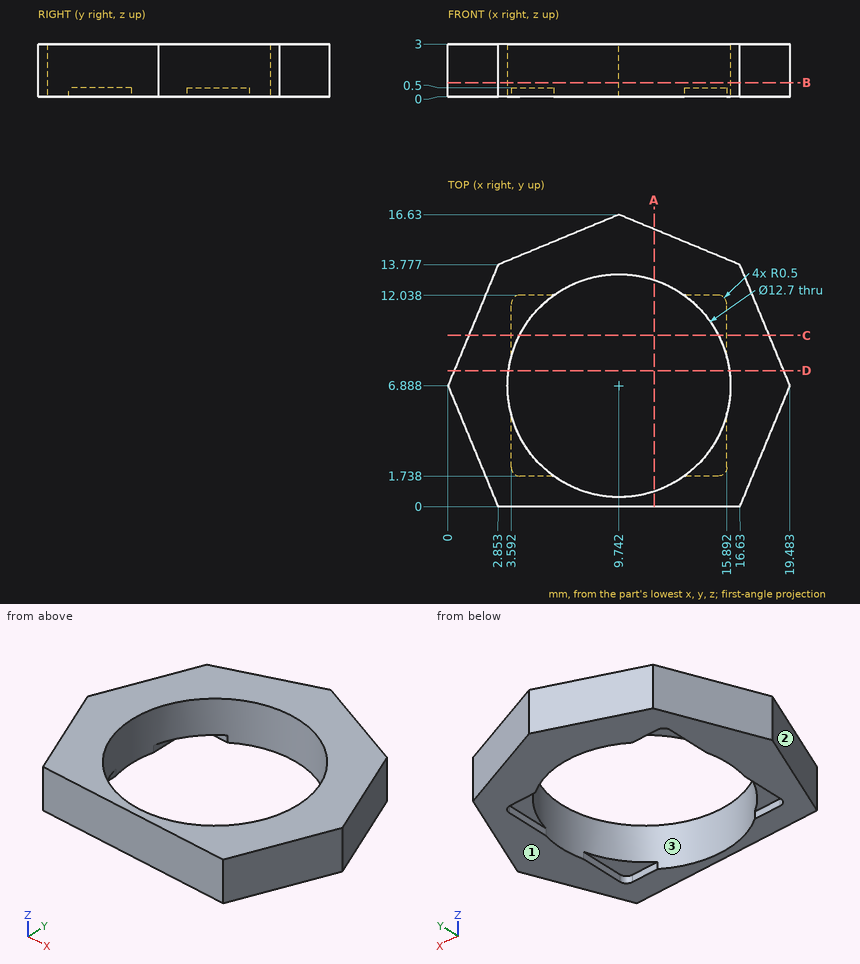
For this review, use the dimensioned drawing (mm, ordinates from the lowest corner) and the shaded views. Give positions to 0.01 mm unless a question says otherwise; leave off trailing zeros. Write each loop counter-clockwise with the first axis right and the second up, starting at its lowest first coordinate (ties: lowest second). Pieces come first, ordered by that corner, then holes. Notation, with made-up numbers: M 46,54.25 L 70,54.25 A8 cw 70,63.25 Z; hole C 45,42.25 d4. An arc over 180 degrees is marked long. Write item = value, one per line. Start each with the question number.
Q1. We need section A-A (x = 11.75). State the section outline as (y, z) points (1 decimal).
Q2. Mouldability with a two-part tool opening along X and no side actions: class the marked faces 1, 2 and 3 as released by +X, released by -X, zero draft, split by the parting line, or undercut.
Q3. For line 1 (X direction, y = 10.5, z = 0.1) (1 decimal); line 2 (X direction, y = 10.25, z = 0.65) (1 decimal); line 3 (Y direction, x = 14.5, z = 1.3) (1 decimal), list the stretches that pass through material, from the lowest coordinate up.
Q4. Clearance check with flat-ended pins moving along their axes: pin 1 (0.7 mm diameter, centred on x = 15, y = 10.5, fed in from -Z); pin 2 (0.6 mm diameter, centred on y = 3.5, z = 0.5, fed in from +X); pin 3 (0.6 mm diameter, centred on x = 5.5, z = 0.5, fed in from +Y). State where each tip first meets the part, or that it passes through.
Q5. We need section D-D (y = 7.75). State the section outline as (x, z) points.
Q6. We need section C-C (y = 9.75). State the section outline as (x, z) points (1 decimal).
Q7. We need section B-B (z = 0.8). State the section outline as (x, y) points, plus the area to 3 significant figures.
Result set:
q1.outline = M 0,0 L 0.9,0 L 0.9,3 L 0,3 Z; M 12.9,0 L 15.8,0 L 15.8,3 L 12.9,3 Z
q2.face_1 = zero draft
q2.face_2 = released by -X
q2.face_3 = undercut
q3.line_1 = 1.5 to 3.6, 15.9 to 18
q3.line_2 = 1.4 to 4.4, 15.1 to 18.1
q3.line_3 = 0 to 2.7, 11.1 to 14.7
q4.pin_1 = 0.5
q4.pin_2 = 18.2
q4.pin_3 = 15
q5.outline = M 0.36,0 L 3.45,0 L 3.45,3 L 0.36,3 Z; M 16.03,0 L 19.13,0 L 19.13,3 L 16.03,3 Z
q6.outline = M 1.2,0 L 3.6,0 L 3.6,0.5 L 4.1,0.5 L 4.1,3 L 1.2,3 Z; M 15.4,0.5 L 15.9,0.5 L 15.9,0 L 18.3,0 L 18.3,3 L 15.4,3 Z
q7.outline = M 0,6.89 L 2.85,0 L 16.63,0 L 19.48,6.89 L 16.63,13.78 L 9.74,16.63 L 2.85,13.78 Z; hole C 9.74,6.89 d12.7
q7.area = 122 mm2
